Autodesk Fusion 360 part; units mm, degrees
sketch "PinWay" plane through (0, 65, 0) normal (0, 1, 0) x (1, 0, 0)
  line L0 (0, 0) -> (0, -30) construction
  line L1 (0, -30) -> (4.125, -30)
  line L2 (4.125, -30) -> (4.125, -25.8571)
  line L3 (-4.125, -30) -> (-4.125, -25.8571)
  line L4 (0, -30) -> (-4.125, -30)
  arc A0 (4.125, -25.8571) -> (-4.125, -25.8571) centre (0, -21.5) ccw
  circle A1 centre (0, -21.5) radius 5.5
  circle A2 centre (0, -21.5) radius 3
  dimension "d1" = 0
  dimension "d2" = 0
  dimension "d3" = 0
  dimension "d4" = 0
  dimension "d5" = 0
  dimension "d6" = 0
extrude "Extrude1" add sketch "PinWay" against normal blind 70 contours A1 | A2
extrude "Extrude2" cut 1 faces at (0.5081, 65, 24.6232) along direction (0, -1, 0) blind 50
chamfer "Chamfer1" distance 0.8 angle 45 1 edges at (-5.1278, 15, 19.5111)
chamfer "Chamfer2" distance 3.2 angle 45 1 edges at (-5.1278, -5, 19.5111)
equation "d150 = BottomPinBlank"
equation "d152 = BottomPinBlank + BottomPinLength"
equation "BottomPinBlank = -70 mm"
equation "BottomPinLength = 20 mm"
equation "d1 = PinWayDiameter"
equation "d2 = PinWayDepth"
equation "d3 = BodyThickness"
equation "d4 = PinWayOpening / 2"
equation "d5 = Pin"
equation "d6 = SpoolPinCenter"
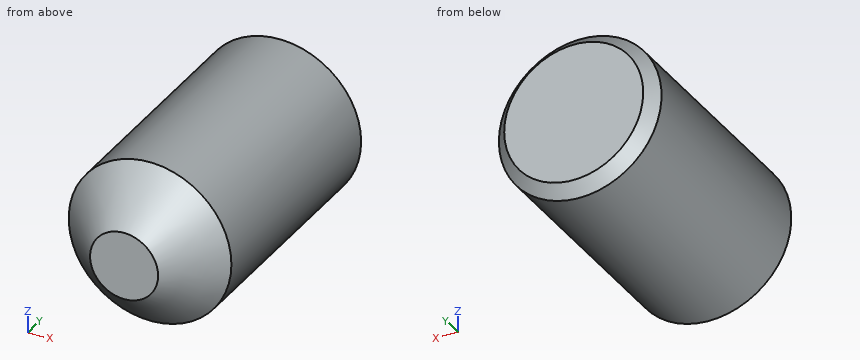
Source: CAD feature listing. Evaluate the final solid. Frame: model axes, mm. Coordinates: 2 decimals unless noted, no trailing zeros. Loops run counter-clockwise (first coordinate to the right, second up) from the corner with the lowest first, then second, coordinate; pieces in that order, holes last. Notation, with made-up numbers: (45, 12) -> (72, 12) arc R18 cw to (72, 18) -> close; hole circle Ø8 at (29, 3). An arc over 180 degrees is marked (long way). One line per item, written item: value. Start each with the question number.
Q1. Contact query for flat-ended pins moving along their axis: P1, Ø2, axis at y = 4, z = 18.5, coming from the -X side; P2, Ø4, axis at y = 1, z = 22, coming from the -X side; P3, Ø1.5, axis at x = 3, y = 12, coming from the +Z side; P4, Ø1, axis at y = 9.5, z = 23.5, coming from the +X side. Output: stop coordinate, or through.
Q2. Section query C-C, the plane y = 13.5. Return the cut outline in (x, z), and give its area (3 significant figures).
Q3. Section query A-A, the plane x = 0. Return the cut outline in (y, z).
Q4. Line query: line 1 along Z through (x, y) = (0.5, -0.25); line 2 along X through (y, z) = (-4, 20.5); line 3 along Y through (x, z) = (2.5, 23.75). Output: solid intervals per line, ascending.
Q5. Section query B-B, the plane z = 21.5. Return the cut outline in (x, y).
Results:
1. P1: x = -5.12
1. P2: x = -5.5
1. P3: z = 26.52
1. P4: x = 5.29
2. outline: circle Ø11 at (0, 21.5)
2. area: 95.0 mm^2
3. outline: (-5, 19.2) -> (-1.8, 16) -> (14.2, 16) -> (15, 16.8) -> (15, 26.2) -> (14.2, 27) -> (-1.8, 27) -> (-5, 23.8) -> close
4. line 1: 16.02 to 26.98
4. line 2: -3.14 to 3.14
4. line 3: -3.94 to 15
5. outline: (-5.5, -1.8) -> (-2.3, -5) -> (2.3, -5) -> (5.5, -1.8) -> (5.5, 14.2) -> (4.7, 15) -> (-4.7, 15) -> (-5.5, 14.2) -> close
